Verification items for the finished model (mm, model axes). A direction names the side the tool comes from. Give positions to 0.01 mm unless a question says otherwise; leave off trailing zeros. Order: outer loops, then holes, each group sorted by start corner. A loop starts at its lowest first (then second) coordinate and runs counter-clockwise, first axis right, second up. Notation, with made-up numbers: (59.25, 22) -> (84.25, 22) arc R14 cw to (84.25, 41) -> close; hole circle Ø3 at (48.25, 88.5). An arc over 180 degrees is marked (long way). Return JSON: item names as keys, results as strings. Group by question number.
(1) Thickness scan on line 1 along Z through (x, y) = (0, -0.25); line 2 along Y through (x, z) = (10, -6); line 3 along Z through (x, y) = (0, -8). Record the ranges inside material, lowest first.
(2) Release check for a two-part mould opening along Z. For faces 3 (the face through (9.139, -1.521, 14.334)), 4 (the face through (6, -12.3, -14)), 5 (the face through (-0.2, -0.6, -6.5)) record: pulls with the +Z half, pulls with the -Z half, needs draft (parallel to the pull), parting line crosses it, or undercut.
(3) Tool access check on faces 1 (the face through (-14.985, -6.368, -0.66)), 2 (the face through (9.139, -9.046, 14.334)). Record the directions out of +Z, -Z, +X, -X, +Y, -Y that give a thin tool (end or side, any length) a straight path to the whole face; none if there is none.
(4) Cross-section at A-A on z = 0. Enter the section's corners in (x, y), then the cut area to 4 significant figures.
(5) Cross-section at C-C on y = -7.5. Enter the section's corners in (x, z), then the cut area to 3 significant figures.
(6) Depth check by flat-ended pin: pin 1 Ø18 at (x, z) = (0, 0) entering from -Y; pin 2 Ø6 at (y, z) = (-6, 4.5) entering from +X; pin 3 Ø6 at (y, z) = (-10, -8.5) entering from +X. Enter the tip coordinate at first touch or a pass-through.
(7) Cross-section at B-B on x = 0. Enter the section's corners in (y, z), then the cut area to 4 significant figures.
Autodesk Fusion 360 part; units mm, degrees
sketch "Sketch1" plane through (0, 0, 0) normal (0, 0, 1) x (1, 0, 0)
  line L0 (0, 0) -> (17, 0)
  line L1 (17, 0) -> (17, -3)
  line L2 (17, -3) -> (17, -5.7)
  line L3 (17, -5.7) -> (17, -12.3)
  line L4 (17, -12.3) -> (15, -12.3)
  line L5 (15, -12.3) -> (15, -0.6)
  line L6 (17, -3) -> (17, -4.35) construction
  line L7 (17, -4.35) -> (16.5, -4.35) construction
  line L8 (17, -3) -> (16.5, -4.35)
  line L9 (16.5, -4.35) -> (17, -5.7)
  line L10 (0, 0) -> (0, -0.6)
  line L11 (0, -0.6) -> (15, -0.6)
  dimension "d1" = 17
  dimension "d2" = 3
  dimension "d4" = 2.7
  dimension "d5" = 6.6
  dimension "d6" = 2
  dimension "d7" = 11.7
  dimension "d8" = 1.35
  dimension "d9" = 0.5
  dimension "d10" = 15
  dimension "d11" = 0.6
  dimension "d12" = 17
revolve "Revolve1" add sketch "Sketch1" angle 360 about axis through (0, 0, 0) along (0, -1, 0) contours L0 L1 L3 L4 L5 L8 L9 L10 L11
sketch "Sketch2" plane through (0, 0, 0) normal (0, 1, 0) x (-1, 0, 0)
  circle A0 centre (0, 0) radius 17
  circle A1 centre (0, 0) radius 16.575
  circle A2 centre (0, 0) radius 6
  dimension "d14" = 34
  dimension "d15" = 33.15
  dimension "d16" = 12
extrude "Extrude1" cut sketch "Sketch2" against normal blind 3 contours A2
equation "d15 = d14 - 0.85 mm"
Verdict:
{
 "1": {"line 1": "-17 to -6, 6 to 17", "line 2": "-0.6 to 0", "line 3": "-17 to -15, 15 to 17"},
 "2": {"face 3": "parting line crosses it", "face 4": "needs draft", "face 5": "undercut"},
 "3": {"face 1": "-Y", "face 2": "+Y, -Y"},
 "4": {"outline": "(-17, -12.3) -> (-15, -12.3) -> (-15, -0.6) -> (-6, -0.6) -> (-6, 0) -> (-17, 0) -> (-17, -3) -> (-16.5, -4.35) -> (-17, -5.7) -> close; (6, -0.6) -> (15, -0.6) -> (15, -12.3) -> (17, -12.3) -> (17, -5.7) -> (16.5, -4.35) -> (17, -3) -> (17, 0) -> (6, 0) -> close", "area": "58.65 mm²"},
 "5": {"outline": "circle Ø34 at (0, 0); hole circle Ø30 at (0, 0)", "area": "201 mm²"},
 "6": {"pin 1": "y = -0.6", "pin 2": "x = 16.93", "pin 3": "x = 16.09"},
 "7": {"outline": "(-12.3, -17) -> (-5.7, -17) -> (-4.35, -16.5) -> (-3, -17) -> (0, -17) -> (0, -6) -> (-0.6, -6) -> (-0.6, -15) -> (-12.3, -15) -> close; (-12.3, 15) -> (-0.6, 15) -> (-0.6, 6) -> (0, 6) -> (0, 17) -> (-3, 17) -> (-4.35, 16.5) -> (-5.7, 17) -> (-12.3, 17) -> close", "area": "58.65 mm²"}
}
